Can you work these out from the drawing? Everything is in mm from the part's minimum corner. Give positions to 0.01 mm unless a question says otherwise; leave off trailing zeros. Order: outer loops, then holes, each group sorted by start corner. A loop starts at its lowest first (then second) coordinate and runs counter-clockwise, first axis right, second up. Notation, with made-up numbers: (-13.5, 32.25) -> (26.5, 32.25) arc R22 cw to (26.5, 40.25) -> close; hole circle Ø6 at (66, 3). An arc over 180 degrees is marked (long way). Answer as CSV lines item,"result". Start each with the question number.
(1) We'd pull the mould along Z, two halves only. Please class the marked faces 1, 2 and 3: released by +Z, released by -Z, zero draft, split by the parting line, or undercut.
(2) Will these pins go through, and if not, where does the flat tip stop? pin 1 Ø3 at (y, z) = (13.5, 6) entering from +X; pin 2 Ø2 at (x, z) = (8, 13.5) entering from -Y; pin 3 Ø2 at (y, z) = (9, 17) entering from +X; pin 4 Ø3 at (y, z) = (3.5, 18) entering from +X.
(3) I need wall thicknesses on L1, parallel to Y at x = 9, z = 10; L2, parallel to Z at x = 3, y = 9.5; L3, parallel to Z at x = 2.5, y = 10. Which ranges of each line are inside material? Lowest first, please.
(4) I want a section at B-B (x = 9). Please give me the cut outline in (y, z).
(5) I want a section at C-C (z = 18). Please give me the cut outline in (x, y), plus the area to 3 significant figures.
(6) I want a section at D-D (x = 2). Please give me the cut outline in (y, z).
(7) I want a section at A-A (y = 9). Please give me the cut outline in (x, z), plus the area to 3 significant figures.
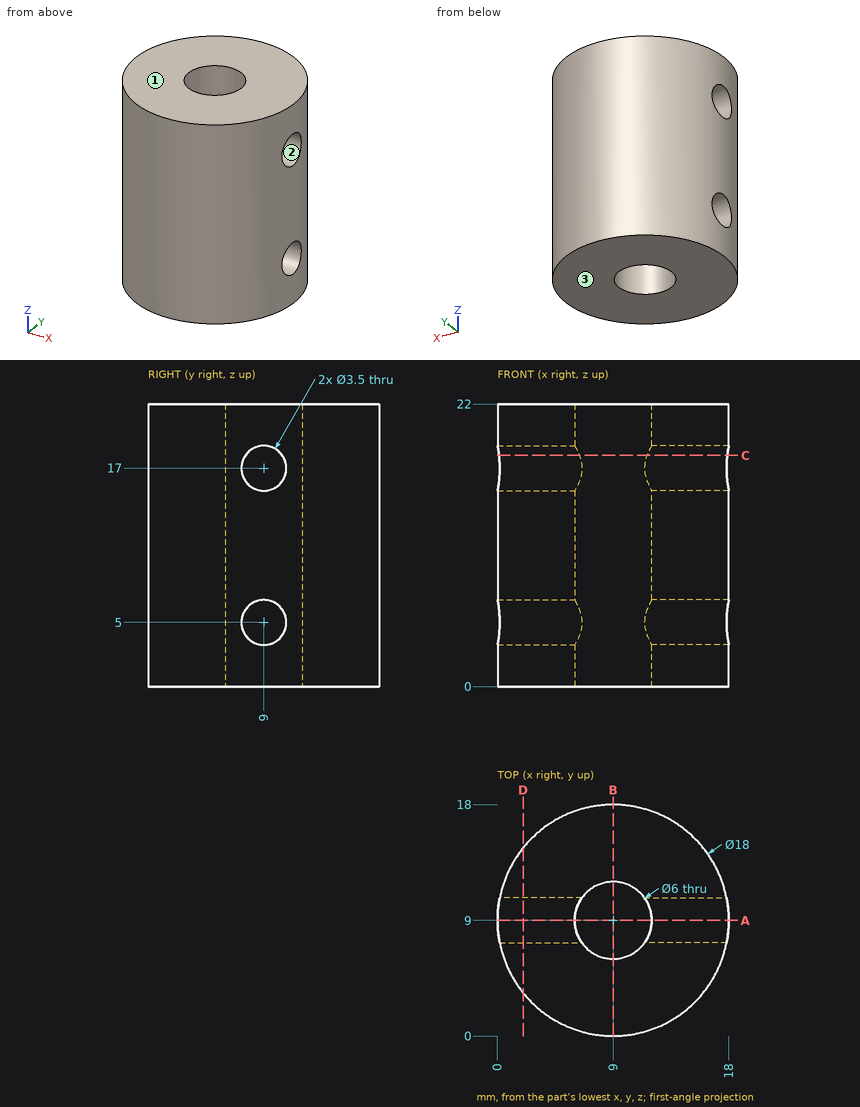
Final values:
1,face 1,"released by +Z"
1,face 2,"undercut"
1,face 3,"released by -Z"
2,pin 1,"x = 17.49"
2,pin 2,"y = 0"
2,pin 3,"through"
2,pin 4,"x = 17.06"
3,L1,"0 to 6, 12 to 18"
3,L2,"0 to 3.32, 6.68 to 15.32, 18.68 to 22"
3,L3,"0 to 3.56, 6.44 to 15.56, 18.44 to 22"
4,outline,"(0, 0) -> (6, 0) -> (6, 22) -> (0, 22) -> close; (12, 0) -> (18, 0) -> (18, 22) -> (12, 22) -> close"
5,outline,"(0.12, 7.56) arc R9 ccw to (17.88, 7.56) -> (11.63, 7.56) arc R3 cw to (6.37, 7.56) -> close; (0.12, 10.44) -> (6.37, 10.44) arc R3 cw to (11.63, 10.44) -> (17.88, 10.44) arc R9 ccw to start"
5,area,"191 mm²"
6,outline,"(3.34, 0) -> (14.66, 0) -> (14.66, 22) -> (3.34, 22) -> close; hole circle Ø3.5 at (9, 5); hole circle Ø3.5 at (9, 17)"
7,outline,"(0, 0) -> (6, 0) -> (6, 3.25) -> (0, 3.25) -> close; (0, 6.75) -> (6, 6.75) -> (6, 15.25) -> (0, 15.25) -> close; (0, 18.75) -> (6, 18.75) -> (6, 22) -> (0, 22) -> close; (12, 0) -> (18, 0) -> (18, 3.25) -> (12, 3.25) -> close; (12, 6.75) -> (18, 6.75) -> (18, 15.25) -> (12, 15.25) -> close; (12, 18.75) -> (18, 18.75) -> (18, 22) -> (12, 22) -> close"
7,area,"180 mm²"
